```python
from build123d import *

# Parameters (mm, degrees)
SKETCH_W        = 126
SKETCH_H        = 140
PAD_DEPTH       = 50
SKETCH002_W     = 120
SKETCH002_H     = 134
POCKET_DEPTH    = 47
SKETCH001_W     = 10
SKETCH001_H     = 14
SKETCH001_W_2   = 3.4
SKETCH001_H_2   = 7.25
PAD001_DEPTH    = 61
SKETCH003_R     = 2.2
POCKET001_DEPTH = 123.001
SKETCH004_R     = 4.5
PAD002_DEPTH    = 5
SKETCH005_R     = 2.2
POCKET002_DEPTH = 8.001


with BuildPart() as part:
    # Sketch → Pad (new body)
    with BuildSketch(Plane.XY):
        Rectangle(SKETCH_W, SKETCH_H)
    extrude(amount=PAD_DEPTH)

    # Sketch002 → Pocket (cut)
    with BuildSketch(Plane.XY.offset(50)):
        Rectangle(SKETCH002_W, SKETCH002_H)
    extrude(amount=-POCKET_DEPTH, mode=Mode.SUBTRACT)

    # Sketch001 → Pad001 (new body)
    with BuildSketch(Plane.XY.offset(3)):
        with Locations((-55, 45)):
            Rectangle(SKETCH001_W, SKETCH001_H)
        with Locations((-55, 45)):
            Rectangle(SKETCH001_W_2, SKETCH001_H_2, mode=Mode.SUBTRACT)
        with Locations((55, 45)):
            Rectangle(SKETCH001_W, SKETCH001_H)
        with Locations((55, 45)):
            Rectangle(SKETCH001_W_2, SKETCH001_H_2, mode=Mode.SUBTRACT)
        with Locations((-55, -45)):
            Rectangle(SKETCH001_W, SKETCH001_H)
        with Locations((-55, -45)):
            Rectangle(SKETCH001_W_2, SKETCH001_H_2, mode=Mode.SUBTRACT)
        with Locations((55, -45)):
            Rectangle(SKETCH001_W, SKETCH001_H)
        with Locations((55, -45)):
            Rectangle(SKETCH001_W_2, SKETCH001_H_2, mode=Mode.SUBTRACT)
    extrude(amount=PAD001_DEPTH)

    # Sketch003 → Pocket001 (cut, through all)
    with BuildSketch(Plane.YZ.offset(60)):
        with Locations((-45, 58)):
            Circle(SKETCH003_R)
        with Locations((45, 58)):
            Circle(SKETCH003_R)
    extrude(amount=-POCKET001_DEPTH, mode=Mode.SUBTRACT)

    # Sketch004 → Pad002 (new body)
    with BuildSketch(Plane.XY.offset(3)):
        with Locations((-38.1655, 50.887)):
            Circle(SKETCH004_R)
        with Locations((38.1655, 50.887)):
            Circle(SKETCH004_R)
        with Locations((-38.1655, -50.887)):
            Circle(SKETCH004_R)
        with Locations((38.1655, -50.887)):
            Circle(SKETCH004_R)
    extrude(amount=PAD002_DEPTH)

    # Sketch005 → Pocket002 (cut, through all)
    with BuildSketch(Plane.XY.offset(8)):
        with Locations((-38.1655, 50.887)):
            Circle(SKETCH005_R)
        with Locations((38.1655, 50.887)):
            Circle(SKETCH005_R)
        with Locations((-38.1655, -50.887)):
            Circle(SKETCH005_R)
        with Locations((38.1655, -50.887)):
            Circle(SKETCH005_R)
    extrude(amount=-POCKET002_DEPTH, mode=Mode.SUBTRACT)


solid = part.part
```
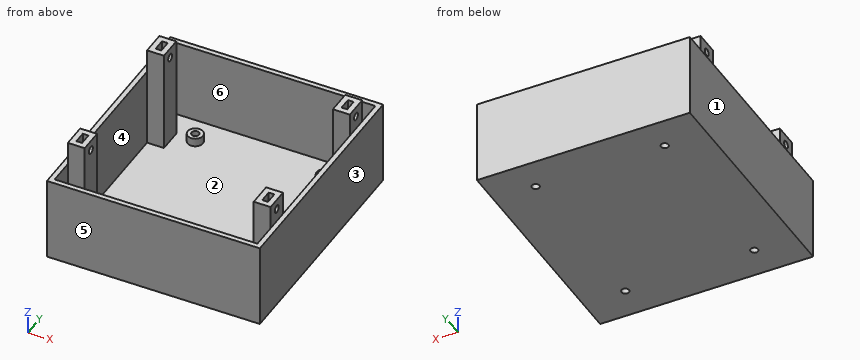
Could you check a few things on this model? Use its own coordinates, in mm. Face numbers are marked on the shaded views. A direction names the side the tool comes from. Coordinates: 2 decimals unless noted, no trailing zeros. Loops run counter-clockwise (first coordinate to the right, second up) from the corner with the lowest first, then second, coordinate; pieces in that order, holes last.
1) Imagine slicing it at A-A (z = 58). State how many separate pieces and enclosed holes the cut face has, and give its area (3 significant figures).
Reported:
separate pieces: 8
enclosed holes: 0
area: 345 mm2
2) Which directions (+Z, -Z, +X, -X, +Y, -Y) give clear straight access to the entire face, cutting with the end or side of a thin tool? Please do the marked faces 5 and 6.
Reported:
face 5: +Z, -Z, +X, -X, -Y
face 6: +Z
3) Thinking about a two-plate mould opening in X: for the marked faces 1, 2, 3 and 4, which applies, released by +X, released by -X, zero draft, split by the parting line, or undercut?
Reported:
face 1: released by -X
face 2: undercut
face 3: released by +X
face 4: undercut
4) Imagine slicing it at B-B (y = 7). List the corners of the cut face in (x, z) for me.
Reported:
outline: (-63, 0) - (63, 0) - (63, 50) - (60, 50) - (60, 3) - (-60, 3) - (-60, 50) - (-63, 50) - close
5) Will these pins go through, and if not, where does the flat tip stop? pin 1 Ø12 at (x, y) = (27.5, -3) entering from +Z; pin 2 Ø7 at (y, z) = (43.5, 58.5) entering from -X; pin 3 Ø4.5 at (x, y) = (-38, -49.5) entering from +Z.
Reported:
pin 1: stops at z = 3
pin 2: stops at x = -60
pin 3: stops at z = 8
6) Imagine slicing it at C-C (x = -20.5). List the corners of the cut face in (y, z) for me, and give its area (3 significant figures).
Reported:
outline: (-70, 0) - (70, 0) - (70, 50) - (67, 50) - (67, 3) - (-67, 3) - (-67, 50) - (-70, 50) - close
area: 702 mm2
7) Please list where these lines run through material, in increasing order: line 1 along X through (y, z) = (43.5, 48); line 2 along Y through (x, z) = (-12, 29); line 3 along Z through (x, y) = (-57.7, -45).
Reported:
line 1: x = -63 to -56.7, -53.3 to -50, 50 to 53.3, 56.7 to 63
line 2: y = -70 to -67, 67 to 70
line 3: z = 0 to 55.8, 60.2 to 64
